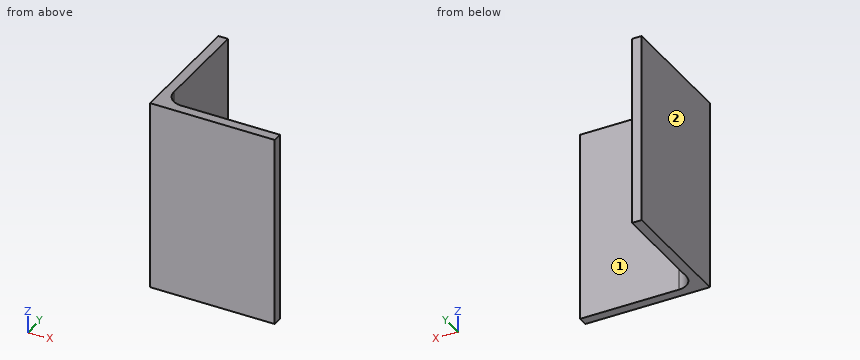
Autodesk Fusion 360 part; units mm, degrees
sketch "スケッチ1" plane through (0, 0, 0) normal (0, 0, 1) x (1, 0, 0)
  line L0 (0, 65) -> (0, 0)
  line L1 (5, 13.5) -> (5, 65)
  line L2 (65, 5) -> (13.5, 5)
  line L3 (0, 0) -> (65, 0)
  arc A0 (5, 13.5) -> (13.5, 5) centre (13.5, 13.5) ccw
  line L4 (65, 0) -> (65, 5)
  line L5 (5, 65) -> (0, 65)
extrude "押し出し1" add sketch "スケッチ1" along normal blind 100
Could you check a few things on this model? Use its own coordinates, in mm. Face numbers are marked on the shaded views. A direction names the side the tool comes from. Give positions to 0.01 mm unless a question says otherwise; leave off trailing zeros. Loops run counter-clockwise (first coordinate to the right, second up) from the corner with the lowest first, then second, coordinate; pieces in that order, holes last. Notation, with made-up numbers: M -6,-26 L -2,-26 A7 ccw -2,-14 Z; hole C 10,77 d11. An arc over 180 degrees is marked long. Answer as a JSON object with one key per item and string values.
Q1. For the marked faces 1 and 2, which set-ups out of +Z, -Z, +X, -X, +Y, -Y let a thin tool reach every point of the face, with its end or its side?
Values found:
{"face 1": "+Z, -Z, +X, +Y", "face 2": "+Z, -Z, -X, +Y, -Y"}
Q2. Suppose I cut it at A-A, the plane z = 92. List the corners of the cut face in (x, y) for me, plus the area to 3 significant figures.
Values found:
{"outline": "M 0,0 L 65,0 L 65,5 L 13.5,5 A8.5 cw 5,13.5 L 5,65 L 0,65 Z", "area": "641 mm²"}
Q3. For P1, Ø4, axis at y = 42.5, z = 36.5, coming from the +X side, with a flat end and sliding along its axis, tell me the tip position at first contact or that it passes through.
Values found:
{"P1": "stops at x = 5"}
Q4. Suppose I cut it at B-B, the plane x = 56. List the corners of the cut face in (y, z) for me.
Values found:
{"outline": "M 0,0 L 5,0 L 5,100 L 0,100 Z"}
Q5. If I drill on probe 1 along X at (y, z) = (53.5, 95.5); probe 2 along Y at (x, z) = (7, 14), over which ranges is the centre line in solid material (lowest first)? Write a range as [from, to].
Values found:
{"probe 1": "x = [0, 5]", "probe 2": "y = [0, 8.02]"}
